from build123d import *

# Parameters (mm, degrees)
ESQUISSE1_W             = 110
ESQUISSE1_H             = 110
BOSS_EXTRU_1_DEPTH      = 4
ESQUISSE2_W             = 110
ESQUISSE2_H             = 100
BOSS_EXTRU_2_DEPTH      = 4
ESQUISSE3_W             = 100
ESQUISSE3_H             = 100
ENL_V_MAT_EXTRU_1_DEPTH = 1
ESQUISSE6_R             = 5
BOSS_EXTRU_3_DEPTH      = 5
NERVURE1_REACH          = 139.095
ESQUISSE8_WALL_W        = 346.189200108
ESQUISSE8_WALL_H        = 4
NERVURE6_REACH          = 139.095
ESQUISSE9_WALL_W        = 346.189200108
ESQUISSE9_WALL_H        = 4


with BuildPart() as part:
    # Esquisse1 → Boss.-Extru.1 (new body)
    with BuildSketch(Plane.XY):
        with Locations((55, 27.788461538)):
            Rectangle(ESQUISSE1_W, ESQUISSE1_H)
    extrude(amount=BOSS_EXTRU_1_DEPTH)

    # Esquisse2 → Boss.-Extru.2 (add)
    with BuildSketch(Plane.XZ.offset(27.211538462)):
        with Locations((55, 4)):
            Rectangle(ESQUISSE2_W, ESQUISSE2_H)
    extrude(amount=BOSS_EXTRU_2_DEPTH)

    # Esquisse3 → Enlèv. mat.-Extru.1 (cut)
    with BuildSketch(Plane(origin=(0, 0, 0), x_dir=(-1, 0, 0), z_dir=(0, 0, -1))):
        with Locations((-55, 27.788461538)):
            Rectangle(ESQUISSE3_W, ESQUISSE3_H)
    extrude(amount=-ENL_V_MAT_EXTRU_1_DEPTH, mode=Mode.SUBTRACT)

    # Esquisse6 → Boss.-Extru.3 (add)
    with BuildSketch(Plane.XZ.offset(31.211538462)):
        with Locations(Location((7, 47, 0), (0, 0, 90))):
            Circle(ESQUISSE6_R)
        with Locations(Location((103, 47, 0), (0, 0, 90))):
            Circle(ESQUISSE6_R)
        with Locations(Location((7, -39, 0), (0, 0, 90))):
            Circle(ESQUISSE6_R)
        with Locations(Location((103, -39, 0), (0, 0, 90))):
            Circle(ESQUISSE6_R)
    extrude(amount=BOSS_EXTRU_3_DEPTH)

    # Esquisse8 wall → Nervure1 (add, up to next)
    with BuildSketch(Plane(origin=(15, -1.607688641, 27.863002208), x_dir=(0, 0.731538566297, -0.681800063083), z_dir=(0, 0.681800063083, 0.731538566297)), mode=Mode.PRIVATE) as nervure1_sk1:
        Rectangle(ESQUISSE8_WALL_W, ESQUISSE8_WALL_H)
    nervure1_tool1 = extrude(nervure1_sk1.sketch, amount=-NERVURE1_REACH, mode=Mode.PRIVATE) - part.part
    add(nervure1_tool1.solids().sort_by_distance((15, -1.607688641, 27.863002208))[0])

    # Esquisse9 wall → Nervure6 (add, up to next)
    with BuildSketch(Plane(origin=(95, -1.607688641, 27.863002208), x_dir=(0, -0.731538566297, 0.681800063083), z_dir=(0, -0.681800063083, -0.731538566297)), mode=Mode.PRIVATE) as nervure6_sk1:
        Rectangle(ESQUISSE9_WALL_W, ESQUISSE9_WALL_H)
    nervure6_tool1 = extrude(nervure6_sk1.sketch, amount=NERVURE6_REACH, mode=Mode.PRIVATE) - part.part
    add(nervure6_tool1.solids().sort_by_distance((95, -1.607688641, 27.863002208))[0])


solid = part.part
Input: part model. Units: mm. Frame: model coordinates. A direction names the side the tool comes from. Coordinates: 2 decimals unless noted, no trailing zeros. Loops run counter-clockwise (first coordinate to the right, second up) from the corner with the lowest first, then second, coordinate; pieces in that order, holes last. Notation, with made-up numbers: (54.5, 7.5) -> (88.5, 7.5) arc R16 cw to (88.5, 29.5) -> close; hole circle Ø8 at (57, 5). An arc over 180 degrees is marked (long way). One line per item, written item: value.
(1) Pin query (flat end, axial travel): pin 1 Ø6 at (x, z) = (79, 24.5) entering from -Y; pin 2 Ø6 at (x, y) = (15.5, 24) entering from -Z; pin 3 Ø24 at (y, z) = (0, 30) entering from +X. Return the tip coordinate at first contact, or that it passes through.
Answer below:
pin 1: stops at y = -31.21
pin 2: stops at z = 1
pin 3: stops at x = 97
(2) Ray query, line 1 along X through (y, z) = (-23.5, 36); line 2 along Y through (x, z) = (80.5, -4.5); line 3 along Z through (x, y) = (102.5, 36.5). Return the intervals inside material, ascending.
Answer below:
line 1: x = 13 to 17, 93 to 97
line 2: y = -31.21 to -27.21
line 3: z = 1 to 4
(3) Set-up query: faces 4 (the face through (54, -31.212, 5)), 5 (the face through (51, -25, 0)), 6 (the face through (13, -11, 18)), 7 (the face through (93, -8, 21)). Return all of +Z, -Z, +X, -X, +Y, -Y with unobstructed straight access to the full face (end or side cutting, diameter ignored); none if empty.
Answer below:
face 4: -Y
face 5: -Z, +X, -X, +Y
face 6: +Z, -X, +Y
face 7: +Z, +Y
(4) Cut plane C-C (y = 72.5). Output: boundary loops of the cut face in (x, z).
Answer below:
outline: (0, 0) -> (5, 0) -> (5, 1) -> (105, 1) -> (105, 0) -> (110, 0) -> (110, 4) -> (0, 4) -> close
(5) Draft query along X for faces 1 (the face through (56, 28, 1)), 2 (the face through (7, -36.212, -39)), 3 (the face through (0, 9.2, 3.8)). Return one class per face: pulls with the +X half, pulls with the -X half, needs draft (parallel to the pull), parting line crosses it, or undercut.
Answer below:
face 1: undercut
face 2: needs draft
face 3: pulls with the -X half
(6) Cut plane A-A (z = -39). Output: boundary loops of the cut face in (x, y), then the cut area to 3 significant figures.
Answer below:
outline: (0, -31.21) -> (2, -31.21) -> (2, -36.21) -> (12, -36.21) -> (12, -31.21) -> (98, -31.21) -> (98, -36.21) -> (108, -36.21) -> (108, -31.21) -> (110, -31.21) -> (110, -27.21) -> (0, -27.21) -> close
area: 540 mm2
(7) Cut plane D-D (x = 7). Output: boundary loops of the cut face in (y, z), then the cut area to 3 significant figures.
Answer below:
outline: (-36.21, -44) -> (-31.21, -44) -> (-31.21, -46) -> (-27.21, -46) -> (-27.21, 0) -> (-22.21, 0) -> (-22.21, 1) -> (77.79, 1) -> (77.79, 0) -> (82.79, 0) -> (82.79, 4) -> (-27.21, 4) -> (-27.21, 54) -> (-31.21, 54) -> (-31.21, 52) -> (-36.21, 52) -> (-36.21, 42) -> (-31.21, 42) -> (-31.21, -34) -> (-36.21, -34) -> close
area: 840 mm2
(8) Cut plane B-B (x = 37). Output: boundary loops of the cut face in (y, z), then the cut area to 3 significant figures.
Answer below:
outline: (-31.21, -46) -> (-27.21, -46) -> (-27.21, 0) -> (-22.21, 0) -> (-22.21, 1) -> (77.79, 1) -> (77.79, 0) -> (82.79, 0) -> (82.79, 4) -> (-27.21, 4) -> (-27.21, 54) -> (-31.21, 54) -> close
area: 740 mm2
